```python
from build123d import *

# Parameters (mm, degrees)
SKETCH1_R           = 3.175
BOSS_EXTRUDE1_DEPTH = 40
SKETCH2_R           = 3.175
SKETCH5_R           = 11
BOSS_EXTRUDE2_DEPTH = 1.5
SKETCH4_R           = 11
SKETCH4_R_2         = 9.652
BOSS_EXTRUDE3_DEPTH = 15
SKETCH6_R           = 3
BOSS_EXTRUDE4_DEPTH = 14
FILLET1_R           = 2
FILLET2_R           = 5


with BuildPart() as part:
    # Sketch1 → Boss-Extrude1 (new body)
    with BuildSketch(Plane(origin=(0, 0, 0), x_dir=(1, 0, 0), z_dir=(0, 1, 0))):
        with Locations(Location((0, 0, 0), (0, 0, 270))):
            Circle(SKETCH1_R)
    extrude(amount=BOSS_EXTRUDE1_DEPTH)

    # Sweep1: sweep along a path in Sketch3
    with BuildLine(Plane.XY) as sweep1_path:
        Line((0, 0), (0, -5))
        ThreePointArc((0, -5), (0.892418328, -9.025438943), (3.402448018, -12.296573321))
        Line((3.402448018, -12.296573321), (11.062892449, -18.724449418))
    # Sketch2 → Sweep1 (sweep)
    with BuildSketch(Plane.XZ):
        Circle(SKETCH2_R)
    sweep(path=sweep1_path.line)

    # Sketch5 → Boss-Extrude2 (add)
    with BuildSketch(Plane(origin=(15.71196326, -13.183902576, 0), x_dir=(0, 0, -1), z_dir=(0.7660444431189796, -0.6427876096865375, 0))):
        with Locations(Location((0, -7.232670233, 0), (0, 0, 90))):
            Circle(SKETCH5_R)
    extrude(amount=BOSS_EXTRUDE2_DEPTH)

    # Sketch4 → Boss-Extrude3 (add)
    with BuildSketch(Plane(origin=(16.861029925, -14.148083991, 0), x_dir=(0, 0, -1), z_dir=(0.7660444431189796, -0.6427876096865375, 0))):
        with Locations(Location((0, -7.232670233, 0), (0, 0, 90))):
            Circle(SKETCH4_R)
        with Locations(Location((0, -7.232670233, 0), (0, 0, 90))):
            Circle(SKETCH4_R_2, mode=Mode.SUBTRACT)
    extrude(amount=BOSS_EXTRUDE3_DEPTH)

    # Sketch6 → Boss-Extrude4 (add)
    with BuildSketch(Plane(origin=(0, 40, 0), x_dir=(1, 0, 0), z_dir=(0, 1, 0))):
        with Locations(Location((0, 0, 0), (0, 0, 270))):
            Circle(SKETCH6_R)
    extrude(amount=BOSS_EXTRUDE4_DEPTH)

    # Fillet1
    # the kernel refuses this fillet: 2 mm, written as the material it adds along each edge
    with BuildSketch(Plane(origin=(0, 40, 0), x_dir=(0, 0, 1), z_dir=(-1, 0, 0))) as fillet1_piece_1:
        with BuildLine():
            CenterArc((5, 0.818153409), FILLET1_R, 180, 24.146847997)
            Line((3, 0.818153409), (2.96, 0.818153409))
            Line((2.96, 0.818153409), (2.96, 0))
            Line((2.96, 0), (3, -0.04))
            ThreePointArc((3, -0.04), (3.0875, -0.04), (3.1385, -0.016363068))
            Line((3.1385, -0.016363068), (3.175, 0))
        make_face()
    revolve(axis=Axis((0, 40, 0), (0, 1, 0)))

    # Fillet2
    fillet2_edges = [part.edges().sort_by_distance(p)[0] for p in [
        (9.022041788, -21.156640524, 0),
    ]]
    fillet(fillet2_edges, radius=FILLET2_R)


solid = part.part
```
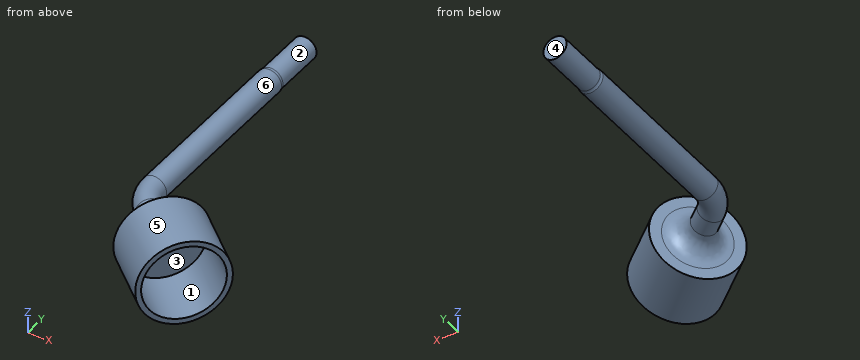
Source: CAD feature listing. Evaluate the final solid. Frame: model axes, mm. Face numbers are marked on the shaded views. A direction names the side the tool comes from. Coordinates: 2 decimals unless noted, no trailing zeros. Write each loop counter-clockwise with the first axis right and the second up, starting at its lowest first coordinate (ties: lowest second). Pieces come first, ordered by that corner, then holes. Notation, with made-up numbers: (49.5, 25) -> (75.5, 25) arc R12 ccw to (75.5, 30) -> close; hole circle Ø10 at (13, 5.25). An arc over 180 degrees is marked (long way). Return JSON: item names as keys, results as strings. Group by question number.
1) Section query B-B, the plane y = 42.5. Return loops of the section in (x, z).
2) Set-up query: the marked faces 5 and 6. Return all of +Z, -Z, +X, -X, +Y, -Y with unobstructed straight access to the full face (end or side cutting, diameter ignored); none if empty.
3) Contact query for flat-ended pins moving along their axis: P1, Ø12, axis at y = 30, z = 8.5, coming from the -X side; P2, Ø4, axis at y = 39, z = -0.5, coming from the +X side (3 decimals); P3, Ø6, axis at x = 19, z = -2, coming from the +Y side; P4, Ø2, axis at x = 1, z = 6, coming from the -Y side. Output: stop coordinate, or through.
4) Ray query, line 1 along Y through (x, z) = (13.5, -1.75); line 2 along X through (y, z) = (-12, -0.75); line 3 along Z through (x, y) = (-1, 26). Return the intervals inside material, ascending.
5) Section query A-A, the plane y = 2.5. Return loops of the section in (x, z) (3 decimals).
6) Mould query, pull axis Y, two halves, no side actions, for the marked faces 1, 2, 3 and 4. Classes: +Y half, -Y half, draft (parallel to the pull), parting line (faces both ways), or undercut.
From the geometry:
{
 "1": {"outline": "circle Ø6 at (0, 0)"},
 "2": {"face 5": "none", "face 6": "+Y"},
 "3": {"P1": "x = -1.96", "P2": "x = 3.175", "P3": "y = -10.3", "P4": "through"},
 "4": {"line 1": "-34.95 to -33.16, -18.15 to -14.33", "line 2": "-0.96 to 7.85, 16.71 to 20.12", "line 3": "-3.01 to 3.01"},
 "5": {"outline": "circle Ø6.35 at (0, 0)"},
 "6": {"face 1": "undercut", "face 2": "draft", "face 3": "undercut", "face 4": "+Y half"}
}
